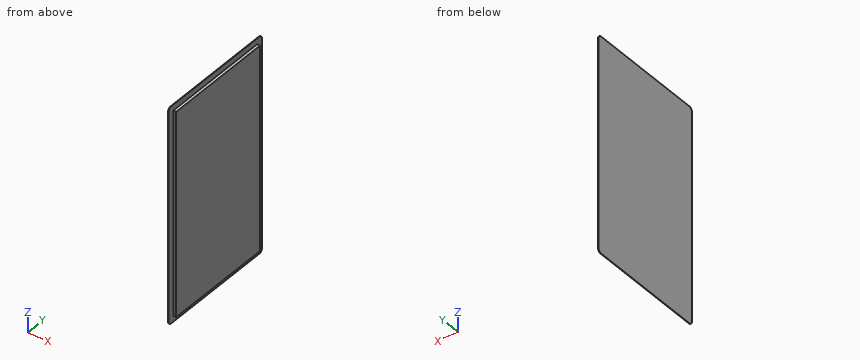
Autodesk Inventor part; units mm, degrees
ref_plane "YZ Plane" through (0, 0, 0) normal (1, 0, 0) x (0, 1, 0)
ref_plane "XZ Plane" through (0, 0, 0) normal (0, 1, 0) x (-1, 0, 0)
ref_plane "XY Plane" through (0, 0, 0) normal (0, 0, 1) x (1, 0, 0)
sketch "Sketch1" plane through (0, 0, 0) normal (1, 0, 0) x (0, 1, 0)
  line L0 (0, 0) -> (110.744, 0)
  line L1 (110.744, 0) -> (110.744, -193.6242)
  line L2 (110.744, -193.6242) -> (0, -193.6242)
  line L3 (0, -193.6242) -> (0, 0)
  dimension "d0" = 193.6242
  dimension "d1" = 110.744
extrude "Extrusion1" add sketch "Sketch1" along normal blind 6.1468
fillet "Fillet1" radius 3.175 4 edges at (3.0734, 110.744, 0) (3.0734, 0, 0) (3.0734, 110.744, -193.6242) (3.0734, 0, -193.6242)
sketch "Sketch3" plane through (6.1468, 0, 0) normal (1, 0, 0) x (0, 0, -1)
  arc A0 (3.175, 110.744) -> (0, 107.569) centre (3.175, 107.569) ccw construction
  arc A1 (190.4492, 0) -> (193.6242, 3.175) centre (190.4492, 3.175) ccw construction
  line L0 (3.175, 107.569) -> (190.4492, 3.175) construction
  arc A2 (193.6242, 107.569) -> (190.4492, 110.744) centre (190.4492, 107.569) ccw construction
  arc A3 (0, 3.175) -> (3.175, 0) centre (3.175, 3.175) ccw construction
  line L1 (190.4492, 107.569) -> (3.175, 3.175) construction
  line L2 (5.1644, 5.6494) -> (188.4598, 5.6494)
  line L3 (188.4598, 5.6494) -> (188.4598, 105.0946)
  line L4 (188.4598, 105.0946) -> (5.1644, 105.0946)
  line L5 (5.1644, 105.0946) -> (5.1644, 5.6494)
  line L6 (5.1644, 5.6494) -> (188.4598, 105.0946) construction
  line L7 (188.4598, 5.6494) -> (5.1644, 105.0946) construction
  arc A4 (190.4492, 0) -> (193.6242, 3.175) centre (190.4492, 3.175) ccw
  line L8 (193.6242, 3.175) -> (193.6242, 107.569)
  arc A5 (193.6242, 107.569) -> (190.4492, 110.744) centre (190.4492, 107.569) ccw
  line L9 (190.4492, 110.744) -> (3.175, 110.744)
  arc A6 (3.175, 110.744) -> (0, 107.569) centre (3.175, 107.569) ccw
  line L10 (0, 107.569) -> (0, 3.175)
  arc A7 (0, 3.175) -> (3.175, 0) centre (3.175, 3.175) ccw
  line L11 (3.175, 0) -> (190.4492, 0)
  point P0 (0, 0)
  point P1 (96.8121, 55.372)
extrude "Extrusion3" cut sketch "Sketch3" against normal blind 2.54
move faces "Move1" translate (3.175, 0, 0) faces at (0, 36.9147, -65.5997)
properties part number "screen"
CAD build for the part. Positions are in the model's coordinates, mm. Give positions to 0.01 mm unless a question says otherwise; leave off trailing zeros. Order: outer loops, then holes, each group sorted by start corner. A loop starts at its lowest first (then second) coordinate and runs counter-clockwise, first axis right, second up. Notation, with made-up numbers: (8.25, -36.5) -> (19.25, -36.5) arc R9 cw to (19.25, -23.5) -> close; hole circle Ø8 at (27, 19). An arc over 180 degrees is marked (long way). Return JSON: item names as keys, results as strings.
Q1. Drill centre lines: line 1 (Z direction, x = 4.65, y = 49); line 2 (Y direction, x = 5.95, z = -79.5). Where is each one in solid material? Low to high.
Working result:
{"line 1": "-188.46 to -5.16", "line 2": "5.65 to 105.09"}
Q2. Saw through at B-B (z = -59). Write the cut outline in (x, y) (3 decimals).
Working result:
{"outline": "(3.175, 0) -> (3.607, 0) -> (3.607, 5.649) -> (6.147, 5.649) -> (6.147, 105.095) -> (3.607, 105.095) -> (3.607, 110.744) -> (3.175, 110.744) -> close"}
Q3. Flat gauge pin, fed straight in: pin 1 (1.5 mm diameter, centred on x = 4.5, y = 41.5, fed in from +Z). Where does the tip first touch, or does it go through?
Working result:
{"pin 1": "z = -5.16"}
Q4. Saw through at C-C (x = 5). Write the cut outline in (y, z).
Working result:
{"outline": "(5.65, -188.46) -> (105.09, -188.46) -> (105.09, -5.16) -> (5.65, -5.16) -> close"}
Q5. Saw through at A-A (y = 77). Write the cut outline in (x, z) (3 decimals).
Working result:
{"outline": "(3.175, -193.624) -> (3.607, -193.624) -> (3.607, -188.46) -> (6.147, -188.46) -> (6.147, -5.164) -> (3.607, -5.164) -> (3.607, 0) -> (3.175, 0) -> close"}
